from build123d import *

# Parameters (mm, degrees)
F1_DEPTH = 38.1
F3_DEPTH = 12.778172


with BuildPart() as f1:
    # F0 (on Top) → F1 (new body)
    with BuildSketch(Plane.XY):
        Polygon((0, 57.923168), (0, 0), (47.275532, 0), (47.275532, 12.777172), (15.474574, 12.777172), (15.474574, 57.923168), align=None)
    extrude(amount=F1_DEPTH)

    # F2 (on face) → F3 (cut, through all)
    with BuildSketch(Plane(origin=(0, 12.777172, 0), x_dir=(-1, 0, 0), z_dir=(0, 1, 0))):
        with BuildLine():
            ThreePointArc((-47.275532, 18.642101), (-43.985861, 30.114338), (-35.116624, 38.1))
            Line((-35.116624, 38.1), (-47.275532, 38.1))
            Line((-47.275532, 38.1), (-47.275532, 18.642101))
        make_face()
        with BuildLine():
            ThreePointArc((-36.633106, 0), (-44.4276, 7.909101), (-47.275532, 18.642101))
            Line((-47.275532, 18.642101), (-47.275532, 0))
            Line((-47.275532, 0), (-36.633106, 0))
        make_face()
    extrude(amount=-F3_DEPTH, mode=Mode.SUBTRACT)


solid = f1.part
CAD build for the part. Positions are in the model's coordinates, mm. A direction names the side the tool comes from. Give positions to 0.01 mm unless a question says otherwise; leave off trailing zeros. Loops run counter-clockwise (first coordinate to the right, second up) from the corner with the lowest first, then second, coordinate; pieces in that order, holes last. Notation, with made-up numbers: M 39,3 L 49,3 A8 ccw 49,15 Z; hole C 10,64 d2. An arc over 180 degrees is marked long. Answer in a Markdown table with one row per item. Add a question column.
Item 1: Band-saw the part on A-A on y = 8. Give the cut face in (x, z), then the cut area to 3 significant figures.
Item 2: Probe probe 1 along Y at (x, z) = (24, 31); probe 2 along X at (y, z) = (35, 17.5); probe 3 along X at (y, z) = (11.5, 33.5). List the from-to ranges inside material, lowest first.
Item 3: Drop flat-ended pins along their axis: P1, Ø8, axis at x = 25, z = 33, coming from the +Y side; P2, Ø2, axis at y = 14, z = 29.5, coming from the +X side. Give the stop position or say it passes through.
Item 4: Tool access for faces 1 (the face through (23, 0, 19)), 2 (the face through (32, 12.777, 19)): list every direction of +Z, -Z, +X, -X, +Y, -Y with a clear straight run to the whole face (end or side of a thin tool).
Item 5: Band-saw the part on C-C on z = 12. Give the cut face in (x, y).
Item 6: Band-saw the part on B-B on x = 24. Give the cut face in (y, z).
Item 7: Band-saw the part on D-D on y = 23.5. Give the cut face in (x, z).
Reply:
| question | item | result |
|---|---|---|
| 1 | outline | M 0,0 L 36.63,0 A21.65 ccw 47.28,18.64 A21.65 ccw 35.12,38.1 L 0,38.1 Z |
| 1 | area | 1,680 mm^2 |
| 2 | probe 1 | y = 0 to 12.78 |
| 2 | probe 2 | x = 0 to 15.47 |
| 2 | probe 3 | x = 0 to 41.37 |
| 3 | P1 | stops at y = 12.78 |
| 3 | P2 | stops at x = 15.47 |
| 4 | face 1 | +Z, -Z, +X, -X, -Y |
| 4 | face 2 | +Z, -Z, +X, +Y |
| 5 | outline | M 0,0 L 46.23,0 L 46.23,12.78 L 15.47,12.78 L 15.47,57.92 L 0,57.92 Z |
| 6 | outline | M 0,0 L 12.78,0 L 12.78,38.1 L 0,38.1 Z |
| 7 | outline | M 0,0 L 15.47,0 L 15.47,38.1 L 0,38.1 Z |
